```python
from build123d import *

# Parameters (mm, degrees)
SKETCH1_W           = 25.4
SKETCH1_H           = 127
BOSS_EXTRUDE1_DEPTH = 146.05
FILLET1_R           = 50.8
SKETCH3_R           = 3.175
SKETCH3_R_2         = 25.019
SKETCH3_R_3         = 2.54
CUT_EXTRUDE1_DEPTH  = 25.4


with BuildPart() as part:
    # Sketch1 → Boss-Extrude1 (new body)
    with BuildSketch(Plane.XY):
        with Locations((12.7, 63.5)):
            Rectangle(SKETCH1_W, SKETCH1_H)
    extrude(amount=BOSS_EXTRUDE1_DEPTH)

    # Fillet1
    fillet1_edges = [part.edges().sort_by_distance(p)[0] for p in [
        (12.7, 127, 0),
        (12.7, 0, 0),
    ]]
    fillet(fillet1_edges, radius=FILLET1_R)

    # Sketch3 → Cut-Extrude1 (cut)
    with BuildSketch(Plane(origin=(25.4, 0, 0), x_dir=(0, 0, -1), z_dir=(1, 0, 0))):
        with Locations((-133.35, 63.5)):
            Circle(SKETCH3_R)
        with Locations((-133.35, 101.6)):
            Circle(SKETCH3_R)
        with Locations((-50.8, 63.5)):
            Circle(SKETCH3_R_2)
        with Locations((-73.914, 86.487)):
            Circle(SKETCH3_R_3)
        with Locations((-27.686, 86.487)):
            Circle(SKETCH3_R_3)
        with Locations((-27.686, 40.513)):
            Circle(SKETCH3_R_3)
        with Locations((-73.914, 40.513)):
            Circle(SKETCH3_R_3)
    extrude(amount=-CUT_EXTRUDE1_DEPTH, mode=Mode.SUBTRACT)


solid = part.part
```
CAD build for the part. Positions are in the model's coordinates, mm. Give positions to 0.01 mm unless a question says otherwise; leave off trailing zeros. Order: outer loops, then holes, each group sorted by start corner. A loop starts at its lowest first (then second) coordinate and runs counter-clockwise, first axis right, second up. Notation, with made-up numbers: M 21,-38.5 L 28,-38.5 A21 ccw 28,-28.5 Z; hole C 71.5,74.25 d5. An arc over 180 degrees is marked long. Put each result on its own line as item: value. Start each with the question number.
(1) Saw through at C-C, the plane x = 14. Write the cut outline in (y, z) (3 decimals).
(2) Saw through at B-B, the plane y = 63.5. Write the cut outline in (x, z) (3 decimals), then the cut area to 3 significant figures.
(3) Saw through at A-A, the plane z = 69. Write the cut outline in (x, y).
(4) Drill centre lines: line 1 along Y through (x, z) = (17.25, 133.35) (3 decimals); line 2 along Z through (x, y) = (16, 103.5); line 3 along Z through (x, y) = (21.5, 69). Where is each one in solid material? Low to high.
(5) Flat gauge pins, fed straight in: pin 1 Ø5.5 at (y, z) = (101.6, 133.35) entering from -X; pin 2 Ø6 at (y, z) = (17.5, 49) entering from -X; pin 3 Ø4 at (x, y) = (17, 33) entering from -Z. Where does each tip first touch, or does it go through?
(6) Saw through at D-D, the plane y = 101.6. Write the cut outline in (x, z) (3 decimals).
Check result:
1. outline: M 0,50.8 A50.8 ccw 50.8,0 L 76.2,0 A50.8 ccw 127,50.8 L 127,146.05 L 0,146.05 Z; hole C 40.513,27.686 d5.08; hole C 40.513,73.914 d5.08; hole C 63.5,50.8 d50.038; hole C 63.5,133.35 d6.35; hole C 86.487,27.686 d5.08; hole C 86.487,73.914 d5.08; hole C 101.6,133.35 d6.35
2. outline: M 0,0 L 25.4,0 L 25.4,25.781 L 0,25.781 Z; M 0,75.819 L 25.4,75.819 L 25.4,130.175 L 0,130.175 Z; M 0,136.525 L 25.4,136.525 L 25.4,146.05 L 0,146.05 Z
2. area: 2,280 mm2
3. outline: M 0,0 L 25.4,0 L 25.4,46.33 L 0,46.33 Z; M 0,80.67 L 25.4,80.67 L 25.4,127 L 0,127 Z
4. line 1: y = 0 to 60.325, 66.675 to 98.425, 104.775 to 127
4. line 2: z = 7.96 to 130.81, 135.89 to 146.05
4. line 3: z = 0 to 26.39, 75.21 to 146.05
5. pin 1: passes through
5. pin 2: stops at x = 0
5. pin 3: stops at z = 2.52
6. outline: M 0,6.806 L 25.4,6.806 L 25.4,130.175 L 0,130.175 Z; M 0,136.525 L 25.4,136.525 L 25.4,146.05 L 0,146.05 Z
